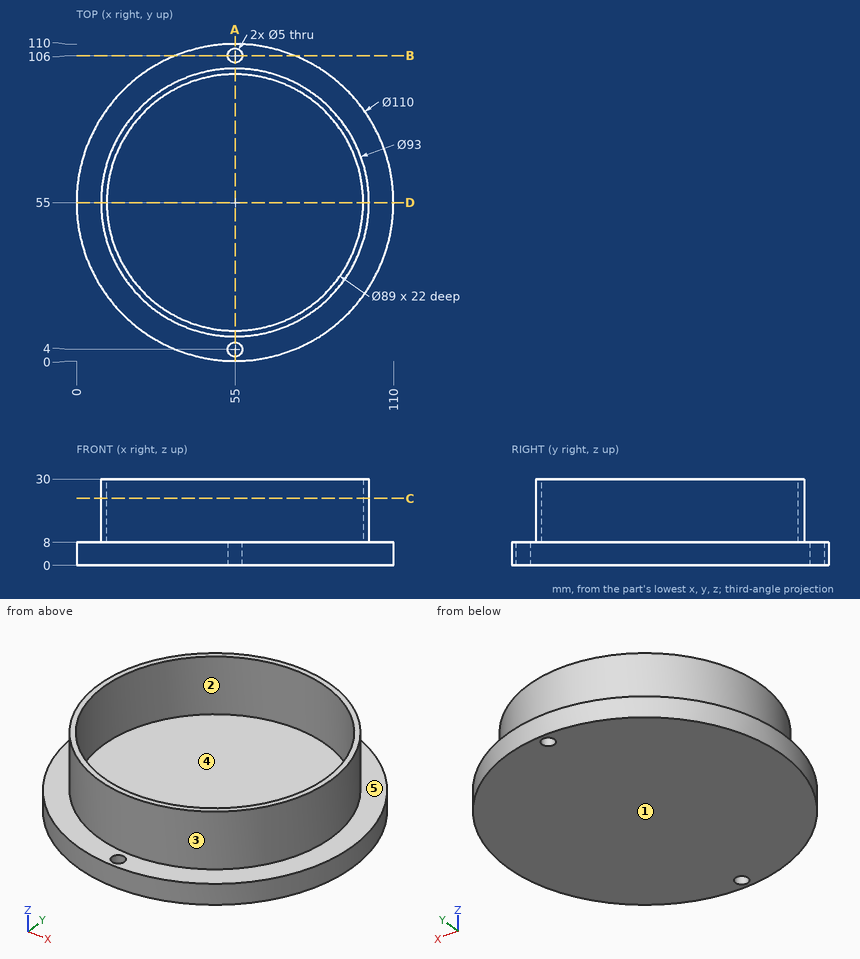
Here's the drawing with two shaded views (mm, measured from the low corner). I have some questions. A direction names the side the tool comes from. Give positions to 0.01 mm unless a question says otherwise; leave off trailing zeros. Write each loop counter-clockwise with the first axis right and the second up, starting at its lowest first coordinate (ties: lowest second). Pieces come first, ordered by that corner, then holes. Notation, with made-up numbers: (6.25, 10) - (31.25, 10) arc R24 ccw to (31.25, 28) - close; hole circle Ø2 at (70.5, -32.75). An arc over 180 degrees is marked (long way). Write item = value, one per line. Start each with the question number.
1. Imagine slicing it at C-C (z = 23.25). Please give me the cut outline in (x, y).
2. Thinking about a two-plate mould opening in Y: for the marked faces 3, 4 and 5, which applies, released by +Y, released by -Y, zero draft, split by the parting line, or undercut?
3. Imagine slicing it at A-A (x = 55). Please give me the cut outline in (y, z).
4. Please list where these lines run through material, in increasing order: line 1 (Y direction, x = 55, z = 3); line 2 (Y direction, x = 55, z = 14.5); line 3 (X direction, y = 56, z = 28).
5. Imagine slicing it at D-D (y = 55). Please give me the cut outline in (x, z).
6. Imagine slicing it at B-B (y = 106). Please give me the cut outline in (x, z), and give its area (3 significant figures).
7. For pin 1 (4 mm diameter, centred on x = 53.5, z = 20, fed in from +Y); pin 2 (6 mm diameter, centred on x = 69, y = 20, fed in from +Z); pin 3 (10 mm diameter, centred on x = 28, z = 16.5, fed in from +Y); pin 4 (2 mm diameter, centred on x = 46, y = 93, fed in from -Z), each with a flat end and sliding along its axis, tell me the tip position at first contact or that it passes through.
8. On a 3-axis mill with a long thin cutter (end or side, diameter ignored), from which of +Z, -Z, +X, -X, +Y, -Y can I reach the whole of each face in a straight line? I mean the marked faces 1 and 2. Say none if no direction works.
Worked answers:
q1.outline = circle Ø93 at (55, 55); hole circle Ø89 at (55, 55)
q2.face_3 = split by the parting line
q2.face_4 = undercut
q2.face_5 = zero draft
q3.outline = (0, 0) - (1.5, 0) - (1.5, 8) - (0, 8) - close; (6.5, 0) - (103.5, 0) - (103.5, 8) - (101.5, 8) - (101.5, 30) - (99.5, 30) - (99.5, 8) - (10.5, 8) - (10.5, 30) - (8.5, 30) - (8.5, 8) - (6.5, 8) - close; (108.5, 0) - (110, 0) - (110, 8) - (108.5, 8) - close
q4.line_1 = 0 to 1.5, 6.5 to 103.5, 108.5 to 110
q4.line_2 = 8.5 to 10.5, 99.5 to 101.5
q4.line_3 = 8.51 to 10.51, 99.49 to 101.49
q5.outline = (0, 0) - (110, 0) - (110, 8) - (101.5, 8) - (101.5, 30) - (99.5, 30) - (99.5, 8) - (10.5, 8) - (10.5, 30) - (8.5, 30) - (8.5, 8) - (0, 8) - close
q6.outline = (34.41, 0) - (52.5, 0) - (52.5, 8) - (34.41, 8) - close; (57.5, 0) - (75.59, 0) - (75.59, 8) - (57.5, 8) - close
q6.area = 289 mm2
q7.pin_1 = 101.5
q7.pin_2 = 8
q7.pin_3 = 95.97
q7.pin_4 = 0
q8.face_1 = -Z, +X, -X, +Y, -Y
q8.face_2 = +Z
